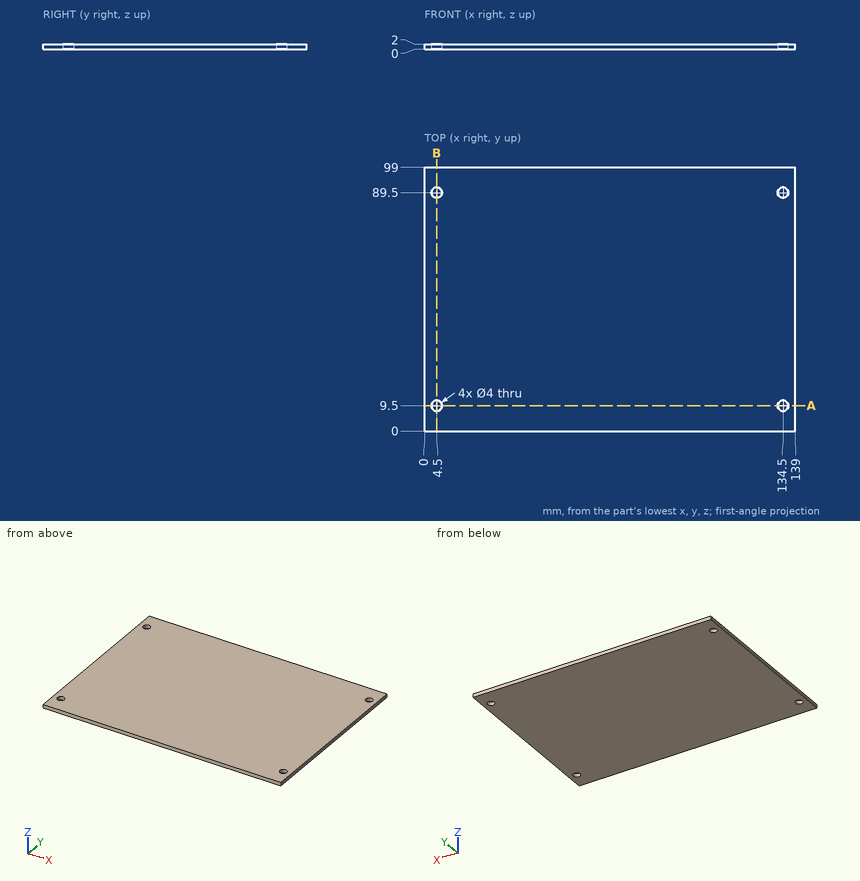
Answer from the drawing. Dimensions are ordinates in mm from the lowest x, y and z of the part. Give positions to 0.01 mm unless a question says otherwise; leave off trailing zeros. Loops run counter-clockwise (first coordinate to the right, second up) from the corner with the lowest first, then second, coordinate; pieces in that order, holes last.
Item 1: The part is cut by section A-A (y = 9.5). Write down the section's boundary in (x, z), and give its area (3 significant figures).
Item 2: The part is cut by section B-B (x = 4.5). Write down the section's boundary in (y, z), and give its area (3 significant figures).
Item 3: This flat-tipped pin is pushed along its axis until it touches: pin 1 Ø3.5 at (x, y) = (4.5, 9.5) entering from -Z. Where does it stop, or does it pass through?
Item 4: Find the intervals of material crossed by line 1 along X through (y, z) = (89.5, 0.55); line 2 along Y through (x, z) = (134.5, 0.9); line 3 along X through (y, z) = (8, 0.65), in increasing order.
Taken from the geometry:
1. outline: (0, 0) - (2.5, 0) - (2.5, 2) - (0, 2) - close; (6.5, 0) - (132.5, 0) - (132.5, 2) - (6.5, 2) - close; (136.5, 0) - (139, 0) - (139, 2) - (136.5, 2) - close
1. area: 262 mm2
2. outline: (0, 0) - (7.5, 0) - (7.5, 2) - (0, 2) - close; (11.5, 0) - (87.5, 0) - (87.5, 2) - (11.5, 2) - close; (91.5, 0) - (99, 0) - (99, 2) - (91.5, 2) - close
2. area: 182 mm2
3. pin 1: passes through
4. line 1: x = 0 to 2.5, 6.5 to 132.5, 136.5 to 139
4. line 2: y = 0 to 7.5, 11.5 to 87.5, 91.5 to 99
4. line 3: x = 0 to 3.18, 5.82 to 133.18, 135.82 to 139
